Build history of the part. All positions in model axes, mm. A direction names the side the tool comes from. Give positions to 0.01 mm unless a question says otherwise; leave off trailing zeros. Write each loop counter-clockwise with the first axis right and the second up, starting at its lowest first coordinate (ties: lowest second). Pieces come first, ordered by that corner, then holes. Notation, with made-up numbers: (4.5, 26) -> (26.5, 26) arc R15 cw to (26.5, 50) -> close; hole circle Ø5 at (-10, 30). An arc over 180 degrees is marked (long way). Write item = value, one per line. Start each with the question number.
Q1. Saw through at A-A, the plane y = -48. List the corners of the cut face in (x, z).
Q2. Saw through at B-B, the plane x = -42. List the corners of the cut face in (y, z), then the cut area to 3 significant figures.
Q3. Mould opens along Y. For faces 1 (the face through (-0.2, -52.3, -14)), 2 (the face through (27, -46, -11)), 3 (the face through (-49.668, -20.595, -10.056)), 4 (the face through (26, -47, -11)) say: pulls with the +Y half, pulls with the -Y half, needs draft (parallel to the pull), parting line crosses it, or undercut.
Q4. Tool access for faces 5 (the face through (49.636, -20.51, -10.056)), 6 (the face through (-27, -46, -11)): list every direction of +Z, -Z, +X, -X, +Y, -Y with a clear straight run to the whole face (end or side of a thin tool).
Q5. Wall check: line 1 (Z direction, x = -24, y = -50); line 2 (X direction, y = -37.5, z = -11); line 3 (X direction, y = -39.6, z = -8.25). Give the ranges that are in metal, low to high.
Q6. Drop flat-ended pins along their axis: P1, Ø4, axis at x = -26, z = -11.5, coming from the +Y side; P2, Ø3, axis at y = -47.5, z = -13, coming from the -X side; P3, Ø3, axis at x = -29.5, z = -12.5, coming from the +Y side. Give the stop position or say it passes through.
Q7. Saw through at D-D, the plane y = -28.5. List the corners of the cut face in (x, z).
Q8. Saw through at C-C, the plane y = -40.5. List the corners of the cut face in (x, z), then the cut area to 3 significant figures.
from build123d import *

# Parameters (mm, degrees)
CYLINDER1548_R               = 59
CYLINDER1548_DEPTH           = 40
CYLINDER1546_R               = 1.5
CYLINDER1546_DEPTH           = 20
CYLINDER1538_R               = 1.5
CYLINDER1538_DEPTH           = 20
CYLINDER1502_R               = 1.5
CYLINDER1502_DEPTH           = 20
CYLINDER1540_R               = 1.5
CYLINDER1540_DEPTH           = 20
BOX540_W                     = 6
BOX540_H                     = 2
BOX540_DEPTH                 = 6
BOX536_W                     = 6
BOX536_H                     = 2
BOX536_DEPTH                 = 6
BOX535_W                     = 6
BOX535_H                     = 2
BOX535_DEPTH                 = 6
BOX539_W                     = 6
BOX539_H                     = 2
BOX539_DEPTH                 = 6
CYLINDER1512_R               = 4
CYLINDER1512_DEPTH           = 20
CYLINDER1512_PLACEMENT_ANGLE = 45
CYLINDER1539_R               = 4
CYLINDER1539_DEPTH           = 20
CYLINDER1539_PLACEMENT_ANGLE = 45
CYLINDER1510_R               = 10
CYLINDER1510_DEPTH           = 40
CYLINDER1541_R               = 10
CYLINDER1541_DEPTH           = 40
CYLINDER1537_R               = 52
CYLINDER1537_DEPTH           = 8
BOX537_W                     = 108
BOX537_H                     = 36
BOX537_DEPTH                 = 8
FILLET024_R                  = 12


with BuildPart() as obj1:
    # Cylinder1548 → Cylinder1548 (new body)
    with BuildSketch(Plane(origin=(0, -17, 13), x_dir=(1, 0, 0), z_dir=(0, -1, 0))):
        Circle(CYLINDER1548_R)
    extrude(amount=CYLINDER1548_DEPTH)


with BuildPart() as obj2:
    # Cylinder1546 → Cylinder1546 (new body)
    with BuildSketch(Plane(origin=(24, -40, -5), x_dir=(1, 0, 0), z_dir=(0, -1, 0))):
        Circle(CYLINDER1546_R)
    extrude(amount=CYLINDER1546_DEPTH)


with BuildPart() as obj3:
    # Cylinder1538 → Cylinder1538 (new body)
    with BuildSketch(Plane(origin=(51, -40, 7), x_dir=(1, 0, 0), z_dir=(0, -1, 0))):
        Circle(CYLINDER1538_R)
    extrude(amount=CYLINDER1538_DEPTH)


with BuildPart() as obj4:
    # Cylinder1502 → Cylinder1502 (new body)
    with BuildSketch(Plane(origin=(-51, -40, 7), x_dir=(1, 0, 0), z_dir=(0, -1, 0))):
        Circle(CYLINDER1502_R)
    extrude(amount=CYLINDER1502_DEPTH)


with BuildPart() as compound912:
    # Cylinder1540 → Cylinder1540 (new body)
    with BuildSketch(Plane(origin=(-24, -40, -5), x_dir=(1, 0, 0), z_dir=(0, -1, 0))):
        Circle(CYLINDER1540_R)
    extrude(amount=CYLINDER1540_DEPTH)

    # Compound912: union obj2, obj3, obj4
    add(obj2.part)
    add(obj3.part)
    add(obj4.part)


with BuildPart() as krychle540:
    # Box540 → Box540 (new body)
    with BuildSketch(Plane(origin=(21, -47, -8), x_dir=(1, 0, 0), z_dir=(0, 0, 1))):
        with Locations((3, 1)):
            Rectangle(BOX540_W, BOX540_H)
    extrude(amount=BOX540_DEPTH)


with BuildPart() as krychle536:
    # Box536 → Box536 (new body)
    with BuildSketch(Plane(origin=(48, -45, 4), x_dir=(1, 0, 0), z_dir=(0, 0, 1))):
        with Locations((3, 1)):
            Rectangle(BOX536_W, BOX536_H)
    extrude(amount=BOX536_DEPTH)


with BuildPart() as krychle535:
    # Box535 → Box535 (new body)
    with BuildSketch(Plane(origin=(-54, -45, 4), x_dir=(1, 0, 0), z_dir=(0, 0, 1))):
        with Locations((3, 1)):
            Rectangle(BOX535_W, BOX535_H)
    extrude(amount=BOX535_DEPTH)


with BuildPart() as compound916:
    # Box539 → Box539 (new body)
    with BuildSketch(Plane(origin=(-27, -47, -8), x_dir=(1, 0, 0), z_dir=(0, 0, 1))):
        with Locations((3, 1)):
            Rectangle(BOX539_W, BOX539_H)
    extrude(amount=BOX539_DEPTH)

    # Compound916: union Krychle540, Krychle536, Krychle535
    add(krychle540.part)
    add(krychle536.part)
    add(krychle535.part)


with BuildPart() as obj5:
    # Cylinder1512 → Cylinder1512 (new body)
    with BuildSketch(Plane.XY):
        Circle(CYLINDER1512_R)
    extrude(amount=CYLINDER1512_DEPTH)


with BuildPart() as obj5_1:
    # Cylinder1512 placement: moved
    add(obj5.part.moved(Location((39.6, -39.6, -10))).rotate(Axis((39.6, -39.6, -10), (0, 0, 1)), CYLINDER1512_PLACEMENT_ANGLE))


with BuildPart() as compound921:
    # Cylinder1539 → Cylinder1539 (new body)
    with BuildSketch(Plane.XY):
        Circle(CYLINDER1539_R)
    extrude(amount=CYLINDER1539_DEPTH)


with BuildPart() as compound921_1:
    # Cylinder1539 placement: moved
    add(compound921.part.moved(Location((-39.6, -39.6, -10))).rotate(Axis((-39.6, -39.6, -10), (0, 0, -1)), CYLINDER1539_PLACEMENT_ANGLE))

    # Compound921: union obj5
    add(obj5_1.part)


with BuildPart() as obj6:
    # Cylinder1510 → Cylinder1510 (new body)
    with BuildSketch(Plane(origin=(-59, -17, 0), x_dir=(1, 0, 0), z_dir=(0, 0, 1))):
        Circle(CYLINDER1510_R)
    extrude(amount=CYLINDER1510_DEPTH)


with BuildPart() as compound919:
    # Cylinder1541 → Cylinder1541 (new body)
    with BuildSketch(Plane(origin=(59, -17, 0), x_dir=(1, 0, 0), z_dir=(0, 0, 1))):
        Circle(CYLINDER1541_R)
    extrude(amount=CYLINDER1541_DEPTH)

    # Compound919: union obj6
    add(obj6.part)


with BuildPart() as obj7:
    # Cylinder1537 → Cylinder1537 (new body)
    with BuildSketch(Plane.XY.offset(20)):
        Circle(CYLINDER1537_R)
    extrude(amount=CYLINDER1537_DEPTH)


with BuildPart() as common006:
    # Box537 → Box537 (new body)
    with BuildSketch(Plane(origin=(-54, -53, 20), x_dir=(1, 0, 0), z_dir=(0, 0, 1))):
        with Locations((54, 18)):
            Rectangle(BOX537_W, BOX537_H)
    extrude(amount=BOX537_DEPTH)

    # Cut548: cut obj7
    add(obj7.part, mode=Mode.SUBTRACT)


with BuildPart() as common006_1:
    # Cut548 placement: moved
    add(common006.part.moved(Location((0, 0, -20))))

    # Cut544: cut Compound919
    add(compound919.part, mode=Mode.SUBTRACT)


with BuildPart() as common006_2:
    # Cut544 placement: moved
    add(common006_1.part.moved(Location((0, 0, -8))))

    # Cut546: cut Compound921
    add(compound921_1.part, mode=Mode.SUBTRACT)

    # Cut547: cut Compound916
    add(compound916.part, mode=Mode.SUBTRACT)

    # Cut545: cut Compound912
    add(compound912.part, mode=Mode.SUBTRACT)

    # Fillet024
    fillet024_edges = [common006_2.edges().sort_by_distance(p)[0] for p in [
        (-54, -25.660254, -4),
        (54, -25.660254, -4),
    ]]
    fillet(fillet024_edges, radius=FILLET024_R)


with BuildPart() as common006_3:
    # Fillet024 placement: moved
    add(common006_2.part.moved(Location((0, 0, -6))))

    # Common006: intersect obj1
    add(obj1.part, mode=Mode.INTERSECT)


solid = common006_3.part
Report:
q1.outline = (-54, -10.77) arc R59 ccw to (-52.46, -14) -> (-20, -14) -> (-20, -6) -> (-54, -6) -> close; (20, -14) -> (52.46, -14) arc R59 ccw to (54, -10.77) -> (54, -6) -> (20, -6) -> close; hole circle Ø3 at (-24, -11); hole circle Ø3 at (24, -11)
q2.outline = (-53, -14) -> (-42.8, -14) -> (-42.8, -6) -> (-53, -6) -> close; (-36.4, -14) -> (-30.66, -14) -> (-30.66, -6) -> (-36.4, -6) -> close
q2.area = 128 mm2
q3.face_1 = needs draft
q3.face_2 = undercut
q3.face_3 = pulls with the +Y half
q3.face_4 = undercut
q4.face_5 = +Z, -Z, +X, +Y
q4.face_6 = -Z
q5.line_1 = -14 to -12.5, -9.5 to -6
q5.line_2 = -53.9 to -43, -36.2 to -36.02, 36.02 to 36.2, 43 to 53.9
q5.line_3 = -54 to -43.6, -35.6 to -33.7, 33.7 to 35.6, 43.6 to 54
q6.P1 = -43.82
q6.P2 = -53.67
q6.P3 = -41.75
q7.outline = (-53.74, -11.34) arc R59 ccw to (-52.46, -14) -> (-43.49, -14) -> (-43.49, -6) -> (-53.74, -6) -> close; (43.49, -14) -> (52.46, -14) arc R59 ccw to (53.74, -11.34) -> (53.74, -6) -> (43.49, -6) -> close
q8.outline = (-54, -10.77) arc R59 ccw to (-52.46, -14) -> (-43.5, -14) -> (-43.5, -6) -> (-54, -6) -> close; (-35.7, -14) -> (-32.62, -14) -> (-32.62, -6) -> (-35.7, -6) -> close; (32.62, -14) -> (35.7, -14) -> (35.7, -6) -> (32.62, -6) -> close; (43.5, -14) -> (52.46, -14) arc R59 ccw to (54, -10.77) -> (54, -6) -> (43.5, -6) -> close
q8.area = 213 mm2
